Geometry: final body of the model. Coordinates: model frame, mm. A direction names the side the tool comes from. Give positions to 0.01 mm unless a question says otherwise; leave off trailing zeros. Write each loop counter-clockwise with the first axis right and the second up, starting at its lowest first coordinate (ties: lowest second). Pieces come first, ordered by that corner, then holes. Notation, with made-up numbers: (-31.75, 11.5) -> (-24.75, 11.5) arc R30 ccw to (-24.75, 33.5) -> close; hole circle Ø11 at (8.25, 52.25). An arc over 180 degrees is marked (long way). Answer as a JSON object with one key per item and string values.
from build123d import *

# Parameters (mm, degrees)
SKETCH2_R           = 3.5
BOSS_EXTRUDE1_DEPTH = 0.5
SKETCH3_R           = 5
BOSS_EXTRUDE2_DEPTH = 1.5
CHAMFER1_SIZE       = 0.4


with BuildPart() as part:
    # Sketch2 → Boss-Extrude1 (new body)
    with BuildSketch(Plane.XY):
        Circle(SKETCH2_R)
    extrude(amount=BOSS_EXTRUDE1_DEPTH)

    # Sketch3 → Boss-Extrude2 (add)
    with BuildSketch(Plane.XY.offset(0.5)):
        Circle(SKETCH3_R)
    extrude(amount=BOSS_EXTRUDE2_DEPTH)

    # Chamfer1
    chamfer1_edges = [part.edges().sort_by_distance(p)[0] for p in [
        (-5, 0, 2),
    ]]
    chamfer(chamfer1_edges, length=CHAMFER1_SIZE)

    # Sketch4 → Cut-Revolve1 (revolve, cut)
    with BuildSketch(Plane(origin=(0, 0, 0), x_dir=(0, -1, 0), z_dir=(1, 0, 0)), mode=Mode.PRIVATE) as cut_revolve1_sk:
        Polygon((3, -2), (0, -2), (0, 0), (1.7, 0), (1.7, -0.7), align=None)
    revolve(cut_revolve1_sk.sketch.rotate(Axis((0, 0, 2), (0, 0, -1)), 90), axis=Axis((0, 0, 2), (0, 0, -1)), mode=Mode.SUBTRACT)


solid = part.part
Q1. Set-up query: faces 1 (the cylindrical face through (0.37, -1.66, 0.35)), 2 (the flat face through (2.2, -3.3, 0.5)). Return all of +Z, -Z, +X, -X, +Y, -Y with unobstructed straight access to the full face (end or side cutting, diameter ignored); none if empty.
Values:
{"face 1": "+Z, -Z", "face 2": "-Z"}
Q2. Material intervals for L1, parallel to Y at x = 0, z = 0.25; L2, parallel to Y at x = 0, z = 0.55; L3, parallel to Z at x = -4, y = -1.25, sorted ascending. Write a range as from..to.
Values:
{"L1": "-3.5..-1.7, 1.7..3.5", "L2": "-5..-1.7, 1.7..5", "L3": "0.5..2"}
Q3. Cut plane D-D (z = 0.3). Return the cut outline in (x, y).
Values:
{"outline": "circle Ø7 at (0, 0); hole circle Ø3.4 at (0, 0)"}
Q4. Cut plane A-A (x = 0). Return the cut outline in (y, z), and give its area (3 significant figures).
Values:
{"outline": "(-5, 0.5) -> (-3.5, 0.5) -> (-3.5, 0) -> (-1.7, 0) -> (-1.7, 0.7) -> (-3, 2) -> (-4.6, 2) -> (-5, 1.6) -> close; (1.7, 0) -> (3.5, 0) -> (3.5, 0.5) -> (5, 0.5) -> (5, 1.6) -> (4.6, 2) -> (3, 2) -> (1.7, 0.7) -> close", "area": "9.85 mm²"}
Q5. Mould query, pull axis X, two halves, no side actions, for faces 3 (the conical face through (0, -2, 1)), 4 (the flat face through (2, 1, 0)), 5 (the cylindrical face through (-1.08, -4.88, 1.04)). Classes: pulls with the +X half, pulls with the -X half, needs draft (parallel to the pull), parting line crosses it, or undercut.
Values:
{"face 3": "undercut", "face 4": "needs draft", "face 5": "parting line crosses it"}
Q6. Cut plane C-C (z = 1.75). Return the cut outline in (x, y).
Values:
{"outline": "circle Ø9.7 at (0, 0); hole circle Ø5.5 at (0, 0)"}
Q7. First-contact query: P1, Ø3, axis at x = -2.5, y = 2, coming from the -Z side; P2, Ø3, axis at x = 0, y = 0, coming from the -Z side; P3, Ø2, axis at x = -1, y = 1, coming from the +Z side. Flat tips, straight axial feed; report the tip coordinate or a pass-through.
Values:
{"P1": "z = 0", "P2": "through", "P3": "z = 1.41"}
